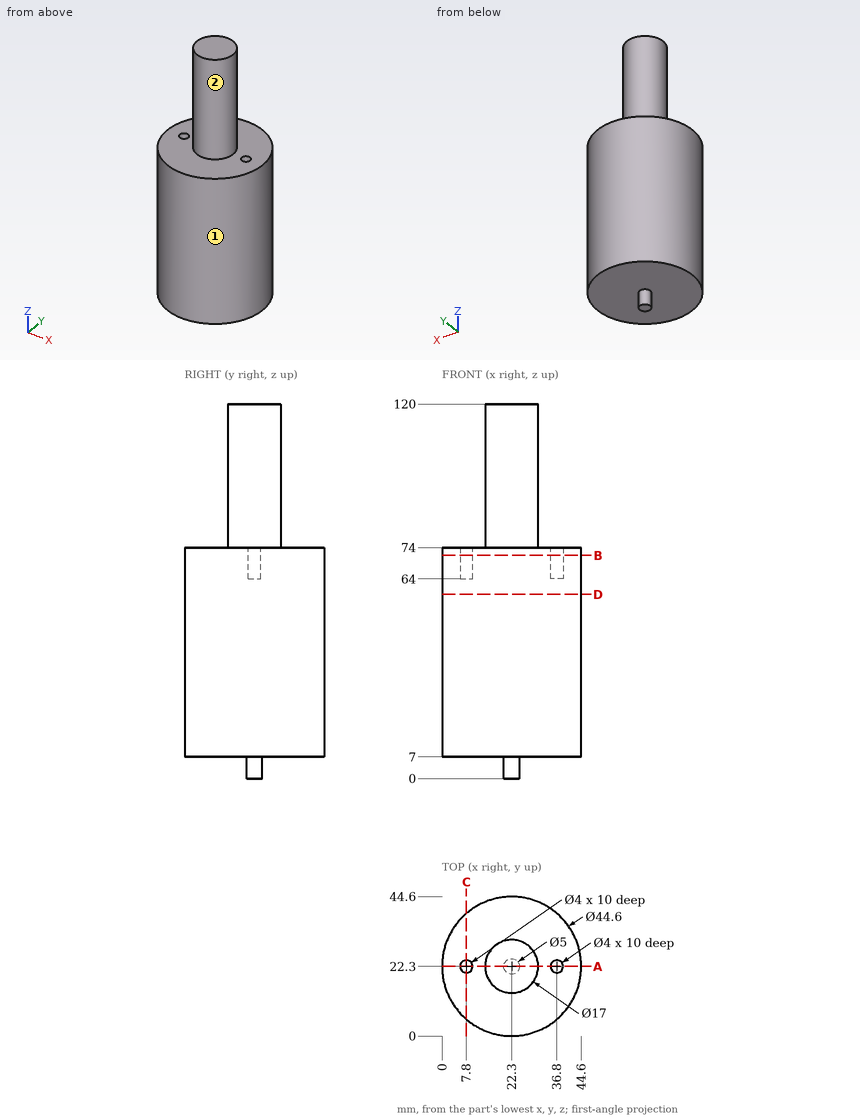
Here's the drawing with two shaded views (mm, measured from the low corner). I have some questions. A direction names the side the tool comes from. Coordinates: 2 decimals unless noted, no trailing zeros. Loops run counter-clockwise (first coordinate to the right, second up) from the corner with the lowest first, then second, coordinate; pieces in that order, holes last. Notation, with made-up numbers: (85.5, -11.75) - (97.5, -11.75) arc R9 ccw to (97.5, -1.75) - close; hole circle Ø7 at (-20.75, 79.5). An arc over 180 degrees is marked (long way). Answer as CSV lines item,"result". Start each with the question number.
1) Suppose I cut it at D-D (z = 59). Please give me the cut outline in (x, y).
2) Which directions (+Z, -Z, +X, -X, +Y, -Y) give clear straight access to the entire face, cutting with the end or side of a thin tool? Please do the marked faces 1 and 2.
3) Suppose I cut it at C-C (x = 7.8). Please give me the cut outline in (y, z), plus the area to 3 significant figures.
4) For pin 1 (6 mm diameter, centred on y = 37, z = 35.5, fed in from +X); pin 2 (12 mm diameter, centred on x = 30.5, z = 13.5, fed in from +Y); pin 3 (2 mm diameter, centred on x = 36.5, y = 22, fed in from +Z), each with a flat end and sliding along its axis, tell me the tip position at first contact or that it passes through.
5) I need wall thicknesses on line 1 (X direction, y = 22, z = 71); line 2 (Z direction, x = 15.5, y = 30.5); line 3 (X direction, y = 21.5, z = 36). Which ranges of each line are inside material? Lowest first, please. Write a range as from..to.
6) Suppose I cut it at A-A (y = 22.3). Please give me the cut outline in (x, z).
7) Suppose I cut it at B-B (z = 71.5). Please give me the cut outline in (x, y).
Check result:
1,outline,"circle Ø44.6 at (22.3, 22.3)"
2,face 1,"+Z, -Z"
2,face 2,"+Z"
3,outline,"(5.36, 7) - (39.24, 7) - (39.24, 74) - (24.3, 74) - (24.3, 64) - (20.3, 64) - (20.3, 74) - (5.36, 74) - close"
3,area,"2,230 mm²"
4,pin 1,"stops at x = 41.28"
4,pin 2,"stops at y = 44.49"
4,pin 3,"stops at z = 64"
5,line 1,"x = 0..5.82, 9.78..34.82, 38.78..44.6"
5,line 2,"z = 7..74"
5,line 3,"x = 0.01..44.59"
6,outline,"(0, 7) - (19.8, 7) - (19.8, 0) - (24.8, 0) - (24.8, 7) - (44.6, 7) - (44.6, 74) - (38.8, 74) - (38.8, 64) - (34.8, 64) - (34.8, 74) - (30.8, 74) - (30.8, 120) - (13.8, 120) - (13.8, 74) - (9.8, 74) - (9.8, 64) - (5.8, 64) - (5.8, 74) - (0, 74) - close"
7,outline,"circle Ø44.6 at (22.3, 22.3); hole circle Ø4 at (7.8, 22.3); hole circle Ø4 at (36.8, 22.3)"
